```python
from build123d import *

# Parameters (mm, degrees)
F1_DEPTH  = 17
F3_DEPTH  = 25
F6_DEPTH  = 25
F8_SIZE   = 3
F9_W      = 25
F9_H      = 10
F10_DEPTH = 4


with BuildPart() as f1:
    # F0 (on Right) → F1 (new body, symmetric)
    with BuildSketch(Plane.YZ):
        Polygon((-70, 0), (0, 0), (0, 70), (-10, 70), (-10, 20), (-20, 10), (-70, 10), align=None)
    extrude(amount=F1_DEPTH, both=True)


with BuildPart() as f3:
    # F2 (on Front) → F3 (new body)
    with BuildSketch(Plane.XZ):
        with BuildLine():
            ThreePointArc((0, 32.5), (-2.5, 30), (0, 27.5))
            Line((0, 27.5), (0, 30))
            Line((0, 30), (0, 32.5))
        make_face()
        with BuildLine():
            Line((0, 30), (0, 27.5))
            ThreePointArc((0, 27.5), (1.767766953, 28.232233047), (2.5, 30))
            ThreePointArc((2.5, 30), (1.767766953, 31.767766953), (0, 32.5))
            Line((0, 32.5), (0, 30))
        make_face()
    extrude(amount=F3_DEPTH)


with BuildPart() as f3b:
    # F2 (on Front) → F3, piece 2 (new body)
    with BuildSketch(Plane.XZ):
        with BuildLine():
            ThreePointArc((2.5, 55), (-1.767766953, 56.767766953), (0, 52.5))
            ThreePointArc((0, 52.5), (1.767766953, 53.232233047), (2.5, 55))
        make_face()
    extrude(amount=F3_DEPTH)


with BuildPart() as f1_1:
    add(f1.part)

    # F4: cut F3b, F3
    add(f3b.part, mode=Mode.SUBTRACT)
    add(f3.part, mode=Mode.SUBTRACT)


with BuildPart() as f6:
    # F5 (on Top) → F6 (new body)
    with BuildSketch(Plane.XY):
        with BuildLine():
            ThreePointArc((2.5, -30), (1.767766953, -28.232233047), (0, -27.5))
            Line((0, -27.5), (0, -30))
            Line((0, -30), (0, -32.5))
            ThreePointArc((0, -32.5), (1.767766953, -31.767766953), (2.5, -30))
        make_face()
        with BuildLine():
            Line((0, -30), (0, -27.5))
            ThreePointArc((0, -27.5), (-2.5, -30), (0, -32.5))
            Line((0, -32.5), (0, -30))
        make_face()
    extrude(amount=F6_DEPTH)


with BuildPart() as f6b:
    # F5 (on Top) → F6, piece 2 (new body)
    with BuildSketch(Plane.XY):
        with BuildLine():
            ThreePointArc((2.5, -55), (1.767766953, -53.232233047), (0, -52.5))
            ThreePointArc((0, -52.5), (-1.767766953, -56.767766953), (2.5, -55))
        make_face()
    extrude(amount=F6_DEPTH)


with BuildPart() as f1_2:
    add(f1_1.part)

    # F7: cut F6, F6b
    add(f6.part, mode=Mode.SUBTRACT)
    add(f6b.part, mode=Mode.SUBTRACT)

    # F8
    f8_edges = [f1_2.edges().sort_by_distance(p)[0] for p in [
        (-2.5, -30, 10),
        (-2.5, -55, 10),
        (0, -10, 32.5),
        (0, -10, 57.5),
    ]]
    chamfer(f8_edges, length=F8_SIZE)



with BuildPart() as f10:
    # F9 (on Right) → F10 (new body, symmetric)
    with BuildSketch(Plane.YZ):
        Polygon((-45, 0), (0, 0), (0, 70), (-10, 70), (-10, 45), (-45, 10), align=None)
        with Locations((-57.5, 5)):
            Rectangle(F9_W, F9_H)
    extrude(amount=F10_DEPTH, both=True)


with BuildPart() as f10_1:
    # F11: moved
    add(f10.part.moved(Location((13, 0, 0))))


with BuildPart() as f1_3:
    add(f1_2.part)

    add(f10_1.part)  # F12 merges F10
    # F12: F10 across plane
    add(f10_1.part.mirror(Plane.YZ))


solid = f1_3.part
```
Here's how the part is built. I have some questions about the finished solid (model axes, mm). A direction names the side the tool comes from. Round coordinates to 2 decimals unless told otherwise and drop trailing zeros. Order: outer loops, then holes, each group sorted by start corner. A loop starts at its lowest first (then second) coordinate and runs counter-clockwise, first axis right, second up. Notation, with made-up numbers: (-33, -17) -> (22, -17) arc R36 cw to (22, 20) -> close; hole circle Ø6 at (3, 47.25). An arc over 180 degrees is marked (long way). Use a Markdown table: item, result. Add a question column.
(1) If we mould it in two halves opening along X, with no side actions, what happens to faces 3 (the face through (13, -27, 28)), 4 (the face through (17, -22, 25)), 5 (the face through (9, -24, 24))? For each: released by +X, released by -X, zero draft, split by the parting line, or undercut.
(2) I need wall thicknesses on line 1 along Y through (x, z) = (0, 5); line 2 along Y through (x, z) = (-1.5, 4.5); line 3 along X through (y, z) = (-55, 1.5). Which ranges of each line are inside material? Lowest first, please.
(3) For pin 1 Ø6 at (x, z) = (0, 55) entering from -Y; pin 2 Ø6 at (x, y) = (-10.5, -55) entering from +Z; pin 3 Ø6.5 at (x, y) = (0, -55) entering from +Z, each with a flat end and sliding along its axis, tell me the tip position at first contact or that it passes through.
(4) Suppose I cut it at C-C, the plane x = 7. Please give me the cut outline in (y, z).
(5) For faces 1 (the face through (0, -70, 5)), 2 (the face through (4, -10, 51)), which set-ups out of +Z, -Z, +X, -X, +Y, -Y let a thin tool reach every point of the face, with its end or its side?
(6) Suppose I cut it at D-D, the plane y = -11. Please give me the cut outline in (x, z), and give its area (3 significant figures).
(7) Suppose I cut it at A-A, the plane z = 6. Please give me the cut outline in (x, y), and give its area (3 significant figures).
(8) Suppose I cut it at B-B, the plane z = 15. Please give me the cut outline in (x, y).
Verdict:
| question | item | result |
|---|---|---|
| 1 | face 3 | zero draft |
| 1 | face 4 | released by +X |
| 1 | face 5 | undercut |
| 2 | line 1 | -70 to -57.5, -52.5 to -32.5, -27.5 to 0 |
| 2 | line 2 | -70 to -57, -53 to -32, -28 to 0 |
| 2 | line 3 | -17 to -2.5, 2.5 to 17 |
| 3 | pin 1 | y = -7.5 |
| 3 | pin 2 | z = 10 |
| 3 | pin 3 | z = 7.75 |
| 4 | outline | (-70, 0) -> (0, 0) -> (0, 70) -> (-10, 70) -> (-10, 20) -> (-20, 10) -> (-70, 10) -> close |
| 5 | face 1 | +Z, -Z, +X, -X, -Y |
| 5 | face 2 | +Z, -Y |
| 6 | outline | (-17, 0) -> (17, 0) -> (17, 44) -> (9, 44) -> (9, 19) -> (-9, 19) -> (-9, 44) -> (-17, 44) -> close |
| 6 | area | 1,050 mm2 |
| 7 | outline | (-17, -70) -> (17, -70) -> (17, 0) -> (-17, 0) -> close; hole circle Ø5 at (0, -55); hole circle Ø5 at (0, -30) |
| 7 | area | 2,340 mm2 |
| 8 | outline | (-17, -40) -> (-9, -40) -> (-9, -15) -> (9, -15) -> (9, -40) -> (17, -40) -> (17, 0) -> (-17, 0) -> close |
